```python
from build123d import *

# Parameters (mm, degrees)
F1_DEPTH = 7
F3_DEPTH = 50.001
F4_R     = 1.75
F5_DEPTH = 2


with BuildPart() as f1:
    # F0 (on Front) → F1 (new body)
    with BuildSketch(Plane.XZ):
        Polygon((27.5, 15), (27.5, 25), (-27.5, 25), (-27.5, -25), align=None)
    extrude(amount=F1_DEPTH)

    # F2 (on face) → F3 (cut, through all)
    with BuildSketch(Plane.XY.offset(25)):
        Polygon((27.5, 0), (-27.5, 0), (27.5, -1.5), align=None)
        Polygon((27.5, -5.5), (-27.5, -7), (27.5, -7), align=None)
    extrude(amount=-F3_DEPTH, mode=Mode.SUBTRACT)

    # F4 (on face) → F5 (cut)
    with BuildSketch(Plane(origin=(0.170328, -6.245355, 0), x_dir=(0.999628, 0.027263, 0), z_dir=(0.027263, -0.999628, 0))):
        with Locations((-7.680617, 10)):
            Circle(F4_R)
    extrude(amount=-F5_DEPTH, mode=Mode.SUBTRACT)


solid = f1.part
```
Input: part model. Units: mm. Frame: model coordinates. Give positions to 0.01 mm unless a question says otherwise; leave off trailing zeros. Loops run counter-clockwise (first coordinate to the right, second up) from the corner with the lowest first, then second, coordinate; pieces in that order, holes last. Notation, with made-up numbers: M 37.5,60 L 93.5,60 A19 ccw 93.5,70 Z; hole C 79,-12 d7. An arc over 180 degrees is marked long. Answer as CSV lines item,"result". Start each with the question number.
1. Section A-A on z = -5. Return loops of the section in (x, y), plus the area to 3 significant figures.
2. Line query: L1, parallel to Z at x = -6.5, y = -6; L2, parallel to X at y = -5, z = -23; L3, parallel to Y at x = -21, z = 5. Output: solid intervals per line, ascending.
3. Section B-B on y = -3.5. Return loops of the section in (x, z).
4. Pin query (flat end, axial travel): P1, Ø6, axis at x = 11.5, z = 0, coming from the +Y side; P2, Ø12, axis at x = 15.5, z = 17, coming from the -Y side; P3, Ø3, axis at x = -5.5, z = -3, coming from the -Y side. Return the tip coordinate at first contact, or that it passes through.
5. Pull-direction query (Z, two-part tool) for faces 1 (the face through (0, -3, 25)), 2 (the face through (-7.762, -5.475, 11.735)), 3 (the face through (0, -3, -5)); classes: released by +Z, released by -Z, zero draft, split by the parting line, or undercut.
Computed values:
1,outline,"M -27.5,-7 L 0,-6.25 L 0,-0.75 L -27.5,0 Z"
1,area,"172 mm²"
2,L1,"z = -9.73 to 8.58, 11.42 to 25"
2,L2,"x = -27.5 to -24.75"
2,L3,"y = -6.82 to -0.18"
3,outline,"M -27.5,-25 L 27.5,15 L 27.5,25 L -27.5,25 Z"
4,P1,"stops at y = -0.99"
4,P2,"stops at y = -5.99"
4,P3,"stops at y = -6.44"
5,face 1,"released by +Z"
5,face 2,"undercut"
5,face 3,"released by -Z"
